The listing builds one solid part. Answer for the finished solid, in the listing's coordinates (mm). A direction names the side the tool comes from. Round coordinates to 2 decimals unless told otherwise and drop trailing zeros. Write each loop counter-clockwise with the first axis right and the second up, starting at its lowest first coordinate (ties: lowest second). Pieces come first, ordered by that corner, then holes. Notation, with made-up numbers: (-32, -20) - (14, -20) arc R16 cw to (14, 8) - close; hole circle Ø6 at (5.25, 80.5). An arc over 180 degrees is marked (long way). Answer in a Markdown table with one row per item.
from build123d import *

# Parameters (mm, degrees)
F0_W     = 3.5
F0_H     = 10
F0_W_2   = 36
F0_H_2   = 24
F1_DEPTH = 3.5
F3_DEPTH = 3.5
F5_DEPTH = 3.5


with BuildPart() as f1:
    # F0 (on Top) → F1 (new body)
    with BuildSketch(Plane.XY):
        Polygon((19.218762, 12.900007), (19.218762, -27.099993), (74.468762, -27.099993), (74.468762, 32.900007), (-76.031238, 32.900007), (-76.031238, -27.099993), (3.218762, -27.099993), (3.218762, 12.900007), align=None)
        with Locations((-0.781238, -12.099993)):
            Rectangle(F0_W, F0_H, mode=Mode.SUBTRACT)
        with Locations((-37.531238, 2.900007)):
            Rectangle(F0_W_2, F0_H_2, mode=Mode.SUBTRACT)
        with Locations((-0.781238, 17.900007)):
            Rectangle(F0_W, F0_H, mode=Mode.SUBTRACT)
        with Locations((45.093762, 2.900007)):
            Rectangle(F0_W_2, F0_H_2, mode=Mode.SUBTRACT)
    extrude(amount=F1_DEPTH)

    # F2 (on face) → F3 (cut)
    with BuildSketch(Plane.YZ.offset(74.468762)):
        Polygon((-27.099993, 3.5), (-27.099993, 0), (-15.099993, 0), (-13.099993, 3.5), align=None)
        Polygon((-7.099993, 3.5), (-5.099993, 0), (10.900007, 0), (12.900007, 3.5), align=None)
        Polygon((18.900007, 3.5), (20.900007, 0), (32.900007, 0), (32.900007, 3.5), align=None)
    extrude(amount=-F3_DEPTH, mode=Mode.SUBTRACT)

    # F4 (on face) → F5 (cut)
    with BuildSketch(Plane(origin=(-76.031238, 0, 0), x_dir=(0, -1, 0), z_dir=(-1, 0, 0))):
        Polygon((27.099993, 3.5), (13.099993, 3.5), (15.099993, 0), (27.099993, 0), align=None)
        Polygon((7.099993, 3.5), (-12.900007, 3.5), (-10.900007, 0), (5.099993, 0), align=None)
        Polygon((-18.900007, 3.5), (-32.900007, 3.5), (-32.900007, 0), (-20.900007, 0), align=None)
    extrude(amount=-F5_DEPTH, mode=Mode.SUBTRACT)


solid = f1.part
(1) Find the intervals of material crossed by line 1 (X direction, y = -1.5, z = 0.35); line 2 (X direction, y = -6.5, z = 0.65); line 3 (X direction, y = -8, z = 3.2), in increasing order.
Checked values:
| item | result |
|---|---|
| line 1 | x = -72.53 to -55.53, -19.53 to 3.22, 19.22 to 27.09, 63.09 to 70.97 |
| line 2 | x = -76.03 to -55.53, -19.53 to 3.22, 19.22 to 27.09, 63.09 to 74.47 |
| line 3 | x = -76.03 to -55.53, -19.53 to -2.53, 0.97 to 3.22, 19.22 to 27.09, 63.09 to 74.47 |
(2) Flat-ended cylindrical pins translate along their axes: pin 1 (1.8 mm diameter, centred on y = 6.5, z = 2.5, fed in from +X); pin 2 (2 mm diameter, centred on y = 3, z = 2.5, fed in from -X); pin 3 (1 mm diameter, centred on x = 9.5, z = 2.5, fed in from -Y). Find the tip coordinate at first contact, or state that the pin passes through.
Checked values:
| item | result |
|---|---|
| pin 1 | stops at x = 70.97 |
| pin 2 | stops at x = -72.53 |
| pin 3 | stops at y = 12.9 |
(3) Section B-B (y = 1) is taken. Give the vertices of the cut face in (x, z).
Checked values:
| item | result |
|---|---|
| outline | (-72.53, 0) - (-55.53, 0) - (-55.53, 3.5) - (-72.53, 3.5) - close; (-19.53, 0) - (3.22, 0) - (3.22, 3.5) - (-19.53, 3.5) - close; (19.22, 0) - (27.09, 0) - (27.09, 3.5) - (19.22, 3.5) - close; (63.09, 0) - (70.97, 0) - (70.97, 3.5) - (63.09, 3.5) - close |
(4) For faces 5 (the flat face through (72.74, -6.11, 1.77)), 6 (the flat face through (-74.31, -6.09, 1.73)), 7 (the flat face through (72.74, -14.11, 1.73)), 8 (the flat face through (11, 12.9, 2)), 9 (the flat face through (-1, -17.1, 2)), determine the directions among +Z, -Z, +X, -X, +Y, -Y from which every point of the face is accessible in a straight line to the end or side of a thin tool.
Checked values:
| item | result |
|---|---|
| face 5 | +Z, +X |
| face 6 | +Z, -X |
| face 7 | +Z, +X, -Y |
| face 8 | +Z, -Z, -Y |
| face 9 | +Z, -Z |
(5) Section A-A (x = -21.5) is taken. Give the vertices of the cut face in (y, z).
Checked values:
| item | result |
|---|---|
| outline | (-27.1, 0) - (-9.1, 0) - (-9.1, 3.5) - (-27.1, 3.5) - close; (14.9, 0) - (32.9, 0) - (32.9, 3.5) - (14.9, 3.5) - close |
(6) Section D-D (x = 10.5) is taken. Give the vertices of the cut face in (y, z).
Checked values:
| item | result |
|---|---|
| outline | (12.9, 0) - (32.9, 0) - (32.9, 3.5) - (12.9, 3.5) - close |
(7) For a pull along X with two mould halves and no side action, classify faces 1 (the flat face through (-76.031, -10, 2)), 2 (the flat face through (19.219, -7, 2)), 3 (the flat face through (0.969, 18, 2)), 4 (the flat face through (-74.31, -14.09, 1.77)) as pulls with the +X half, pulls with the -X half, needs draft (parallel to the pull), parting line crosses it, or undercut.
Checked values:
| item | result |
|---|---|
| face 1 | pulls with the -X half |
| face 2 | undercut |
| face 3 | undercut |
| face 4 | needs draft |
(8) Section C-C (y = -22) is taken. Give the vertices of the cut face in (x, z), and give its area (3 significant figures).
Checked values:
| item | result |
|---|---|
| outline | (-72.53, 0) - (3.22, 0) - (3.22, 3.5) - (-72.53, 3.5) - close; (19.22, 0) - (70.97, 0) - (70.97, 3.5) - (19.22, 3.5) - close |
| area | 446 mm2 |
